Geometry check sheet. Reference: the model listing, model coordinates, mm. A direction names the side the tool comes from. Give positions to 0.01 mm unless a question says otherwise; leave off trailing zeros. Write each loop counter-clockwise with the first axis right and the second up, starting at its lowest first coordinate (ties: lowest second). Pieces come first, ordered by that corner, then holes. Notation, with made-up numbers: (-30, 74) -> (6, 74) arc R5 cw to (6, 81) -> close; hole circle Ø10 at (63, 55). An arc over 180 degrees is marked (long way). Use a Markdown table: item, result. Add a question column.
from build123d import *

# Parameters (mm, degrees)
BOSS_EXTRUDE1_DEPTH       = 110
F_5_0MM_DOWEL_HOLE1_D     = 5
F_5_0MM_DOWEL_HOLE2_D     = 5
F_5_0MM_DOWEL_HOLE2_DEPTH = 12


with BuildPart() as part:
    # Sketch1 → Boss-Extrude1 (new body)
    with BuildSketch(Plane.XY):
        Polygon((-74.4140625, 0), (75.5859375, 0), (75.5859375, 20), (55.5859375, 20), (55.5859375, 12), (35.5859375, 12), (35.5859375, 20), (-24.4140625, 20), (-24.4140625, 12), (-44.4140625, 12), (-44.4140625, 20), (-74.4140625, 20), align=None)
    extrude(amount=BOSS_EXTRUDE1_DEPTH)

    # Ø5.0mm Dowel Hole1 (through all)
    with Locations(Plane(origin=(-59.4140625, 20, 20), x_dir=(1, 0, 0), z_dir=(0, 1, 0))):
        with Locations((0, 0), (0, -70), (125, 0), (125, -70)):
            Hole(F_5_0MM_DOWEL_HOLE1_D / 2)

    # Ø5.0mm Dowel Hole2
    with Locations(Plane(origin=(-34.4140625, 12, 15), x_dir=(1, 0, 0), z_dir=(0, 1, 0))):
        with Locations((0, 0), (0, -80), (80, 0), (80, -80)):
            Hole(F_5_0MM_DOWEL_HOLE2_D / 2, depth=F_5_0MM_DOWEL_HOLE2_DEPTH)


solid = part.part
1) Sectioned sample at B-B, the plane z = 20. Enter the section's corners in (x, y).
2) Sectioned sample at D-D, the plane x = 38. Enter the section's corners in (y, z).
3) Sectioned sample at A-A, the plane y = 14.5. Enter the section's corners in (x, z), and give its area (3 significant figures).
4) Tool access check on faces 1 (the face through (66, 20, 54)), 2 (the face through (-34, 12, 54)). Record the directions out of +Z, -Z, +X, -X, +Y, -Y that give a thin tool (end or side, any length) a straight path to the whole face; none if there is none.
5) Draft check along Z on faces 3 (the face through (-44.414, 16, 54)), 4 (the face through (64.242, 9.86, 17.892)), 5 (the face through (0, 10, 0)). Enter one of: +Z half, -Z half, draft (parallel to the pull), parting line (faces both ways), or undercut.
6) Sectioned sample at C-C, the plane z = 54. Enter the section's corners in (x, y), and give its area (3 significant figures).
7) Gauge pin test, flat end, axial feed: P1, Ø3, axis at x = 45.59, z = 15, coming from the +Y side. Record the tip position at first contact, or that the pin passes through.
8) Material ranges on probe 1 along X at (y, z) = (15, 5.5); probe 2 along X at (y, z) = (9.25, 90); probe 3 along Z at (x, y) = (46, 3.25), recorded low to high. Write a range as [from, to].
Check values:
| question | item | result |
|---|---|---|
| 1 | outline | (-74.41, 0) -> (-61.91, 0) -> (-61.91, 20) -> (-74.41, 20) -> close; (-56.91, 0) -> (63.09, 0) -> (63.09, 20) -> (55.59, 20) -> (55.59, 12) -> (35.59, 12) -> (35.59, 20) -> (-24.41, 20) -> (-24.41, 12) -> (-44.41, 12) -> (-44.41, 20) -> (-56.91, 20) -> close; (68.09, 0) -> (75.59, 0) -> (75.59, 20) -> (68.09, 20) -> close |
| 2 | outline | (0, 0) -> (12, 0) -> (12, 110) -> (0, 110) -> close |
| 3 | outline | (-74.41, 0) -> (-44.41, 0) -> (-44.41, 110) -> (-74.41, 110) -> close; (-24.41, 0) -> (35.59, 0) -> (35.59, 110) -> (-24.41, 110) -> close; (55.59, 0) -> (75.59, 0) -> (75.59, 110) -> (55.59, 110) -> close; hole circle Ø5 at (-59.41, 20); hole circle Ø5 at (-59.41, 90); hole circle Ø5 at (65.59, 20); hole circle Ø5 at (65.59, 90) |
| 3 | area | 12,000 mm² |
| 4 | face 1 | +Z, -Z, +X, -X, +Y |
| 4 | face 2 | +Z, -Z, +Y |
| 5 | face 3 | draft |
| 5 | face 4 | undercut |
| 5 | face 5 | -Z half |
| 6 | outline | (-74.41, 0) -> (75.59, 0) -> (75.59, 20) -> (55.59, 20) -> (55.59, 12) -> (35.59, 12) -> (35.59, 20) -> (-24.41, 20) -> (-24.41, 12) -> (-44.41, 12) -> (-44.41, 20) -> (-74.41, 20) -> close |
| 6 | area | 2,680 mm² |
| 7 | P1 | through |
| 8 | probe 1 | [-74.41, -44.41], [-24.41, 35.59], [55.59, 75.59] |
| 8 | probe 2 | [-74.41, -61.91], [-56.91, 63.09], [68.09, 75.59] |
| 8 | probe 3 | [0, 12.53], [17.47, 92.53], [97.47, 110] |
